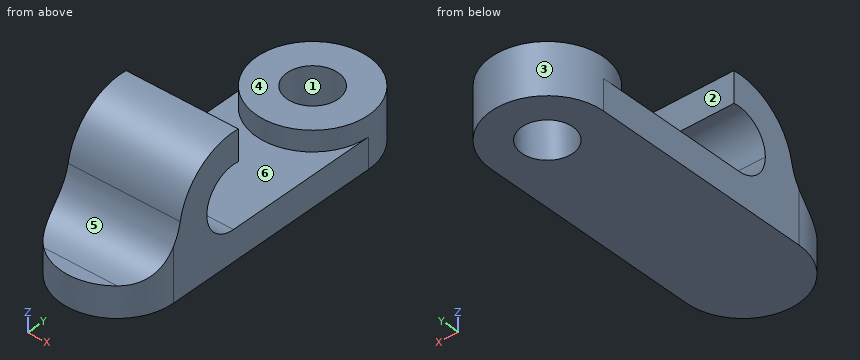
from build123d import *

# Parameters (mm, degrees)
F1_DEPTH = 3
F2_DEPTH = 5
F4_DEPTH = 11
F5_R     = 5


with BuildPart() as f1:
    # F0 (on Top) → F1 (new body)
    with BuildSketch(Plane.XY):
        with BuildLine():
            Line((-5.5, 11), (-5.5, -11))
            ThreePointArc((-5.5, -11), (0, -5.5), (5.5, -11))
            Line((5.5, -11), (5.5, 11))
            ThreePointArc((5.5, 11), (0, 5.5), (-5.5, 11))
        make_face()
        with BuildLine():
            ThreePointArc((5.5, -11), (0, -5.5), (-5.5, -11))
            Line((-5.5, -11), (5.5, -11))
        make_face()
        with BuildLine():
            Line((5.5, -11), (-5.5, -11))
            ThreePointArc((-5.5, -11), (0, -16.5), (5.5, -11))
        make_face()
    extrude(amount=F1_DEPTH)

    # F0 (on Top) → F2 (join)
    with BuildSketch(Plane.XY):
        with BuildLine():
            Line((-2.5, 11), (-5.5, 11))
            ThreePointArc((-5.5, 11), (0, 5.5), (5.5, 11))
            Line((5.5, 11), (2.5, 11))
            ThreePointArc((2.5, 11), (0, 8.5), (-2.5, 11))
        make_face()
        with BuildLine():
            ThreePointArc((5.5, 11), (0, 16.5), (-5.5, 11))
            Line((-5.5, 11), (-2.5, 11))
            ThreePointArc((-2.5, 11), (0, 13.5), (2.5, 11))
            Line((2.5, 11), (5.5, 11))
        make_face()
    extrude(amount=F2_DEPTH)

    # F3 (on face) → F4 (join)
    with BuildSketch(Plane(origin=(-5.5, 0, 0), x_dir=(0, -1, 0), z_dir=(-1, 0, 0))):
        with BuildLine():
            ThreePointArc((3.6959245331, 8.9510570469), (6.1566711465, 8.3042419241), (7.2356117629, 6))
            ThreePointArc((7.2356117629, 6), (6.3569321064, 3.8786796564), (4.2356117629, 3))
            Line((4.2356117629, 3), (9.5210892795, 3))
            ThreePointArc((9.5210892795, 3), (9.3640881698, 9.2761960602), (3.6959245331, 11.975678848))
            Line((3.6959245331, 11.975678848), (3.6959245331, 8.9510570469))
        make_face()
    extrude(amount=-F4_DEPTH)

    # F5
    f5_edges = [f1.edges().sort_by_distance(p)[0] for p in [
        (0, -9.521089, 3),
    ]]
    fillet(f5_edges, radius=F5_R)


solid = f1.part
Work out the finished part from the listing and answer in its coordinate system (mm). Face numbers are marked on the shaded views. A direction names the side the tool comes from. Coordinates: 2 decimals unless noted, no trailing zeros. Loops run counter-clockwise (first coordinate to the right, second up) from the corner with the lowest first, then second, coordinate; pieces in that order, holes last. Notation, with made-up numbers: (-21, 13.25) -> (27, 13.25) arc R19 ccw to (27, 35.25) -> close; hole circle Ø5 at (-12.5, -11). An arc over 180 degrees is marked (long way). Write each question's results on one line, items separated by ' | '. Start each with the question number.
1) Flat-ended cylindrical pins translate along their axes: P1, Ø5.5, axis at x = -1.5, y = 12.5, coming from the +Z side; P2, Ø0.9, axis at x = 1.5, z = 11, coming from the +Y side; P3, Ø2, axis at x = 2, y = -1.5, coming from the +Z side. Find the tip coordinate at first contact, or state that the pin passes through.
2) Consider line 1 along Y through (x, z) = (0, 3.95); line 2 along Y through (x, z) = (0, 3.55); line 3 along Y through (x, z) = (0, 1.1). Determine where each line is inside the solid, lowest interval first.
3) The mould has two halves that part along Y. Classify the marked faces 4, 5 and 6: pulls with the +Y half, pulls with the -Y half, needs draft (parallel to the pull), parting line crosses it, or undercut.
4) Find section A-A on x = 0. Determine the outline of the cut face in (y, z).
5) Find section C-C on y = -5. Determine the outline of the cut face in (x, z).
6) Find section B-B on z = 2.5. Determine the outline of the cut face in (x, y), then the cut area to 3 significant figures.
7) For the marked faces 1, 2 and 3, determine the directions among +Z, -Z, +X, -X, +Y, -Y from which every point of the face is accessible in a straight line to the end or side of a thin tool.
8) Find section D-D on y = 14.5. Determine the outline of the cut face in (x, z).
Response values:
1) P1: stops at z = 5 | P2: stops at y = -3.7 | P3: stops at z = 3
2) line 1: y = -12.22 to -6.43, 5.5 to 8.5, 13.5 to 16.5 | line 2: y = -12.87 to -5.97, 5.5 to 8.5, 13.5 to 16.5 | line 3: y = -16.5 to 8.5, 13.5 to 16.5
3) face 4: needs draft | face 5: pulls with the -Y half | face 6: undercut
4) outline: (-16.5, 0) -> (8.5, 0) -> (8.5, 5) -> (5.5, 5) -> (5.5, 3) -> (-4.24, 3) arc R3 cw (long way) to (-3.7, 8.95) -> (-3.7, 11.98) arc R6 ccw to (-10.23, 7.1) arc R5 cw to (-15.15, 3) -> (-16.5, 3) -> close; (13.5, 0) -> (16.5, 0) -> (16.5, 5) -> (13.5, 5) -> close
5) outline: (-5.5, 0) -> (5.5, 0) -> (5.5, 3.1) -> (-5.5, 3.1) -> close; (-5.5, 8.9) -> (5.5, 8.9) -> (5.5, 11.97) -> (-5.5, 11.97) -> close
6) outline: (-5.5, -11) arc R5.5 ccw to (5.5, -11) -> (5.5, 11) arc R5.5 ccw to (-5.5, 11) -> close; hole circle Ø5 at (0, 11) | area: 317 mm^2
7) face 1: +Z, -Z | face 2: +Z, +X, -X, +Y | face 3: +Z
8) outline: (-4.24, 0) -> (4.24, 0) -> (4.24, 5) -> (-4.24, 5) -> close
